For this review, take the finished solid that the model builds, in its own axes (mm). A direction names the side the tool comes from. Coordinates: 2 decimals unless noted, no trailing zeros. Order: outer loops, then holes, each group sorted by start corner. A loop starts at its lowest first (then second) coordinate and runs counter-clockwise, first axis right, second up. Notation, with made-up numbers: (7.25, 37) - (56.25, 37) arc R9 cw to (56.25, 41) - close; hole circle Ø5 at (-24.5, 26.25). An arc over 180 degrees is marked (long way). One line per item, written item: value. Start each with the question number.
(1) Consider section A-A on z = -21.5. Write out the cut boundary in (x, y) (3 decimals).
(2) For faces 5 (the cylindrical face through (-0.69, -3.1, 30.21)), 6 (the flat face through (0, 0, 40.005)), 7 (the flat face through (19, -10, -16.891)), 8 (the flat face through (19, -10, 16.891)), list the 3-axis set-ups (+Z, -Z, +X, -X, +Y, -Y) from which the entire face can be reached by the end or side of a thin tool; tool diameter is ignored.
(3) To check wall thickness, follow line 1 along Z through (x, y) = (2, -4) (3 decimals); line 2 along X through (y, z) = (10, 33.5); line 3 along Y through (x, z) = (-0.5, -19). State the ranges of each line that lie inside material, in increasing order.
(4) Consider section B-B on z = 10. Write out the cut boundary in (x, y), then the cut area to 3 significant figures.
(5) Mouldability with a two-part tool opening along Z and no side actions: class faces 1 (the cylindrical face through (-2.728, -20.777, -28.912)), 2 (the cylindrical face through (-1.124, 8.563, 26.64)), 3 (the flat face through (2, 3, 31.623)), 4 (the flat face through (0, 0, -41.275)) as released by +Z, released by -Z, zero draft, split by the parting line, or undercut.
(6) Clearance check with flat-ended pins moving along their axes: pin 1 (8 mm diameter, centred on y = -10, z = 25, fed in from -X); pin 2 (1 mm diameter, centred on y = -15.5, z = -5, fed in from +X); pin 3 (10 mm diameter, centred on y = -8, z = -4, fed in from +X). State where each tip first meets the part, or that it passes through.
```python
from build123d import *

# Parameters (mm, degrees)
SKETCH1_R           = 22.86
BOSS_EXTRUDE1_DEPTH = 16.891
SKETCH2_R           = 20.955
BOSS_EXTRUDE2_DEPTH = 24.384
BOSS_EXTRUDE3_START = 7.62
SKETCH3_R           = 20.955
BOSS_EXTRUDE3_DEPTH = 7.62
SKETCH4_R           = 8.636
BOSS_EXTRUDE4_DEPTH = 4.318
FILLET1_R           = 2.54
SKETCH5_R           = 3.175
BOSS_EXTRUDE6_DEPTH = 11.176
SKETCH6_R           = 8.89
BOSS_EXTRUDE7_DEPTH = 8.382
SKETCH7_RX          = 2.54
SKETCH7_RY          = 0.762
BOSS_EXTRUDE8_DEPTH = 8.382
CIRPATTERN1_COUNT   = 21


with BuildPart() as part:
    # Sketch1 → Boss-Extrude1 (new, symmetric)
    with BuildSketch(Plane.XY):
        Circle(SKETCH1_R)
    extrude(amount=BOSS_EXTRUDE1_DEPTH, both=True)

    # Sketch2 → Boss-Extrude2 (add)
    with BuildSketch(Plane(origin=(0, 0, -16.891), x_dir=(-1, 0, 0), z_dir=(0, 0, -1))):
        with Locations(Location((0, 0, 0), (0, 0, 180))):
            Circle(SKETCH2_R)
    extrude(amount=BOSS_EXTRUDE2_DEPTH)

    # Sketch3 → Boss-Extrude3 (add)
    with BuildSketch(Plane.XY.offset(16.891).offset(BOSS_EXTRUDE3_START)):
        Circle(SKETCH3_R)
    extrude(amount=-BOSS_EXTRUDE3_DEPTH)

    # Sketch4 → Boss-Extrude4 (add)
    with BuildSketch(Plane.XY.offset(24.511)):
        Circle(SKETCH4_R)
    extrude(amount=BOSS_EXTRUDE4_DEPTH)

    # Fillet1
    fillet1_edges = [part.edges().sort_by_distance(p)[0] for p in [
        (-20.955, 0, 24.511),
    ]]
    fillet(fillet1_edges, radius=FILLET1_R)

    # Sketch5 → Boss-Extrude6 (add)
    with BuildSketch(Plane.XY.offset(28.829)):
        Circle(SKETCH5_R)
    extrude(amount=BOSS_EXTRUDE6_DEPTH)

    # Sketch6 → Boss-Extrude7 (add)
    with BuildSketch(Plane.XY.offset(40.005)):
        Circle(SKETCH6_R)
    extrude(amount=-BOSS_EXTRUDE7_DEPTH)

    # Sketch7 → Boss-Extrude8 (add)
    with BuildSketch(Plane.XY.offset(40.005)):
        with Locations(Location((0, 8.89), (0, 0, 90))):
            Ellipse(SKETCH7_RX, SKETCH7_RY)
    boss_extrude8 = extrude(amount=-BOSS_EXTRUDE8_DEPTH)

    # CirPattern1: Boss-Extrude8 ×21 about axis
    cirpattern1_axis = Axis((0, 0, 44.069), (0, 0, -1))
    for i in range(1, CIRPATTERN1_COUNT):
        add(boss_extrude8.rotate(cirpattern1_axis, i * 360 / CIRPATTERN1_COUNT))


solid = part.part
```
Geometry check:
1. outline: circle Ø41.91 at (0, 0)
2. face 5: none
2. face 6: +Z, +X, -X, +Y, -Y
2. face 7: -Z
2. face 8: +Z
3. line 1: z = -41.275 to 28.829, 31.623 to 40.005
3. line 2: x = -3.66 to -2.41, -0.69 to 0.69, 2.41 to 3.66
3. line 3: y = -20.95 to 20.95
4. outline: circle Ø45.72 at (0, 0)
4. area: 1,640 mm^2
5. face 1: zero draft
5. face 2: undercut
5. face 3: undercut
5. face 4: released by -Z
6. pin 1: stops at x = -19.74
6. pin 2: stops at x = 17.25
6. pin 3: stops at x = 22.66
